Geometry check sheet. Reference: drawing and pictorial views, mm from the part's lowest x, y, z. A direction names the side the tool comes from. Round coordinates to 2 decimals unless told otherwise and drop trailing zeros. Order: outer loops, then holes, each group sorted by start corner. A loop starts at its lowest first (then second) coordinate and runs counter-clockwise, first axis right, second up.
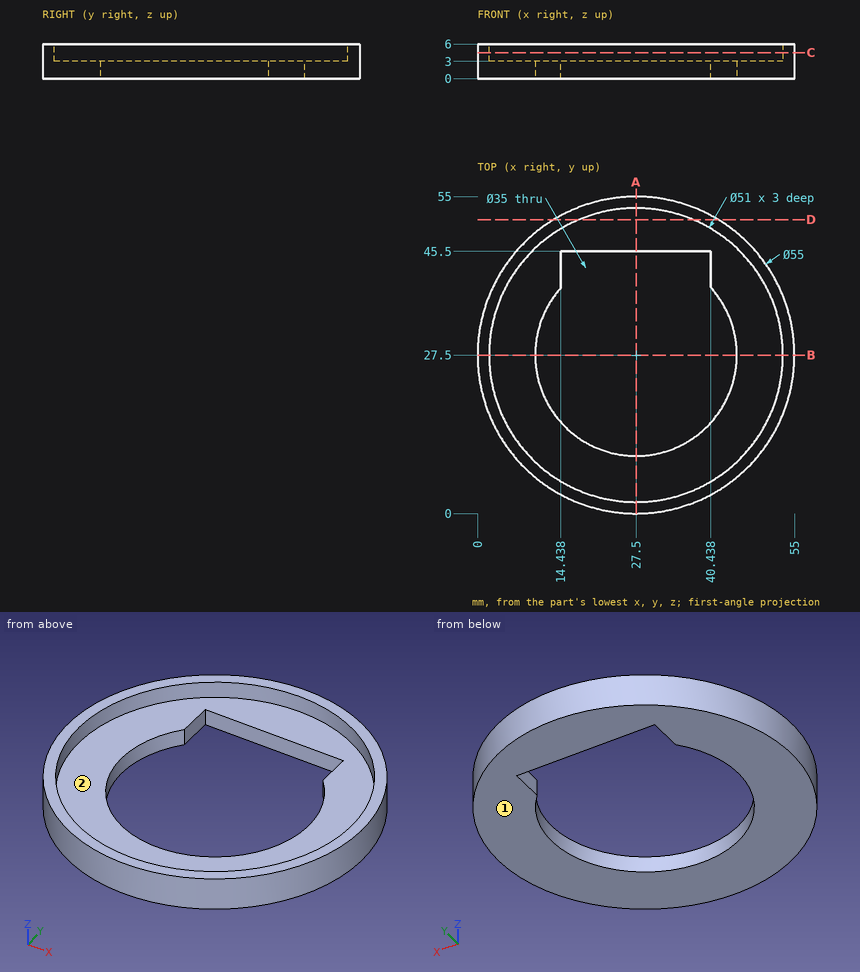
1) Sectioned sample at A-A on x = 27.5. Record the cut outline in (y, z), then the cut area to 3 significant figures.
2) Sectioned sample at C-C on z = 4.5. Record the cut outline in (x, y), then the cut area to 3 significant figures.
3) Sectioned sample at B-B on y = 27.5. Record the cut outline in (x, z).
4) Sectioned sample at D-D on y = 51. Record the cut outline in (x, z).
5) Scan lines: probe 1 along X at (y, z) = (27, 4.5) (1 decimal); probe 2 along Y at (x, z) = (27.5, 2.35). Record each from-to range of solid material in increasing order.
6) Tool access check on the marked faces 1 and 2. Record the directions out of +Z, -Z, +X, -X, +Y, -Y that give a thin tool (end or side, any length) a straight path to the whole face; none if there is none.
7) Go/stop test with flat-tipped pins: pin 1 Ø3.5 at (y, z) = (41.5, 1) entering from +X; pin 2 Ø5 at (x, y) = (47, 33.5) entering from +Z; pin 3 Ø12 at (x, y) = (39.5, 37) entering from -Z; pin 4 Ø12 at (x, y) = (24, 21) entering from -Z. Record where each tip stops, or that it passes through.
Returned:
1. outline: (0, 0) - (10, 0) - (10, 3) - (2, 3) - (2, 6) - (0, 6) - close; (45.5, 0) - (55, 0) - (55, 6) - (53, 6) - (53, 3) - (45.5, 3) - close
1. area: 70.5 mm2
2. outline: circle Ø55 at (27.5, 27.5); hole circle Ø51 at (27.5, 27.5)
2. area: 333 mm2
3. outline: (0, 0) - (10, 0) - (10, 3) - (2, 3) - (2, 6) - (0, 6) - close; (45, 0) - (55, 0) - (55, 6) - (53, 6) - (53, 3) - (45, 3) - close
4. outline: (13.22, 0) - (41.78, 0) - (41.78, 6) - (37.4, 6) - (37.4, 3) - (17.6, 3) - (17.6, 6) - (13.22, 6) - close
5. probe 1: x = 0 to 2, 53 to 55
5. probe 2: y = 0 to 10, 45.5 to 55
6. face 1: -Z, +X, -X, +Y, -Y
6. face 2: +Z
7. pin 1: stops at x = 52.12
7. pin 2: stops at z = 3
7. pin 3: stops at z = 0
7. pin 4: passes through
